```python
from build123d import *

# Parameters (mm, degrees)
CROQUIS1_W              = 50
CROQUIS1_H              = 46
CROQUIS1_W_2            = 44
CROQUIS1_H_2            = 40
SALIENTE_EXTRUIR1_DEPTH = 15
CROQUIS4_W              = 44
CROQUIS4_H              = 3
SALIENTE_EXTRUIR3_DEPTH = 10.7
CORTAR_EXTRUIR1_REACH   = 72.608
CROQUIS7_W              = 3
CROQUIS7_H              = 10.7
SALIENTE_EXTRUIR4_DEPTH = 10.7
SALIENTE_EXTRUIR5_DEPTH = 10.7
CORTAR_EXTRUIR2_REACH   = 72.778
CROQUIS9_R              = 6.65
CORTAR_EXTRUIR3_REACH   = 70.691
CROQUIS10_R             = 6.65
CROQUIS11_W             = 50
CROQUIS11_H             = 31.2
SALIENTE_EXTRUIR6_DEPTH = 2
CROQUIS12_W             = 3
CROQUIS12_H             = 12
SALIENTE_EXTRUIR7_DEPTH = 44
CORTAR_EXTRUIR4_REACH   = 62.537
CROQUIS13_R             = 2.5
REDONDEO1_R             = 2
CROQUIS15_W             = 2
CROQUIS15_H             = 10.7
SALIENTE_EXTRUIR8_DEPTH = 3
CROQUIS16_W             = 2.1
CROQUIS16_H             = 3.3
CORTAR_EXTRUIR5_DEPTH   = 50
CROQUIS17_W             = 2
CROQUIS17_H             = 10.7
SALIENTE_EXTRUIR9_DEPTH = 3
CORTAR_EXTRUIR6_REACH   = 69.968
CROQUIS18_W             = 4.444444444
CROQUIS18_H             = 21.2


with BuildPart() as part:
    # Croquis1 → Saliente-Extruir1 (new body)
    with BuildSketch(Plane(origin=(0, 0, 0), x_dir=(1, 0, 0), z_dir=(0, 1, 0))):
        with Locations((-22, -20)):
            Rectangle(CROQUIS1_W, CROQUIS1_H)
        with Locations((-22, -20)):
            Rectangle(CROQUIS1_W_2, CROQUIS1_H_2, mode=Mode.SUBTRACT)
    extrude(amount=SALIENTE_EXTRUIR1_DEPTH)

    # Croquis4 → Saliente-Extruir3 (add)
    with BuildSketch(Plane(origin=(0, 15, 0), x_dir=(1, 0, 0), z_dir=(0, 1, 0))):
        with Locations((-22, -41.5)):
            Rectangle(CROQUIS4_W, CROQUIS4_H)
    extrude(amount=SALIENTE_EXTRUIR3_DEPTH)

    # Croquis6 → Cortar-Extruir1 (cut, up to next)
    with BuildSketch(Plane.XY.offset(43), mode=Mode.PRIVATE) as cortar_extruir1_sk1:
        Polygon((-22, 24.7), (-11.85, 24.7), (-11.85, 16.7), (-32.15, 16.7), (-32.15, 24.7), align=None)
    cortar_extruir1_tool1 = extrude(cortar_extruir1_sk1.sketch, amount=-CORTAR_EXTRUIR1_REACH, mode=Mode.PRIVATE) & part.part
    add(cortar_extruir1_tool1.solids().sort_by_distance((-22, 20.7, 43))[0], mode=Mode.SUBTRACT)

    # Croquis7 → Saliente-Extruir4 (add)
    with BuildSketch(Plane.XY.offset(43)):
        with Locations((-45.5, 20.35)):
            Rectangle(CROQUIS7_W, CROQUIS7_H)
        with Locations((1.5, 20.35)):
            Rectangle(CROQUIS7_W, CROQUIS7_H)
    extrude(amount=-SALIENTE_EXTRUIR4_DEPTH)

    # Croquis8 → Saliente-Extruir5 (add)
    with BuildSketch(Plane(origin=(0, 15, 0), x_dir=(1, 0, 0), z_dir=(0, 1, 0))):
        Polygon((-47, -28.2), (-44, -28.2), (-44, 0), (0, 0), (0, -28.2), (3, -28.2), (3, 3), (-47, 3), align=None)
    extrude(amount=SALIENTE_EXTRUIR5_DEPTH)

    # Croquis9 → Cortar-Extruir2 (cut, up to next)
    with BuildSketch(Plane.ZY.offset(47), mode=Mode.PRIVATE) as cortar_extruir2_sk1:
        with Locations((7, 15.7)):
            Circle(CROQUIS9_R)
    cortar_extruir2_tool1 = extrude(cortar_extruir2_sk1.sketch, amount=-CORTAR_EXTRUIR2_REACH, mode=Mode.PRIVATE) & part.part
    add(cortar_extruir2_tool1.solids().sort_by_distance((-47, 15.7, 7))[0], mode=Mode.SUBTRACT)

    # Croquis10 → Cortar-Extruir3 (cut, up to next)
    with BuildSketch(Plane.ZY, mode=Mode.PRIVATE) as cortar_extruir3_sk1:
        with Locations((7, 15.7)):
            Circle(CROQUIS10_R)
    cortar_extruir3_tool1 = extrude(cortar_extruir3_sk1.sketch, amount=-CORTAR_EXTRUIR3_REACH, mode=Mode.PRIVATE) & part.part
    add(cortar_extruir3_tool1.solids().sort_by_distance((0, 15.7, 7))[0], mode=Mode.SUBTRACT)

    # Croquis11 → Saliente-Extruir6 (add)
    with BuildSketch(Plane(origin=(0, 25.7, 0), x_dir=(1, 0, 0), z_dir=(0, 1, 0))):
        with Locations((-22, -12.6)):
            Rectangle(CROQUIS11_W, CROQUIS11_H)
    extrude(amount=-SALIENTE_EXTRUIR6_DEPTH)

    # Croquis12 → Saliente-Extruir7 (add)
    with BuildSketch(Plane.ZY):
        with Locations((26.7, 17.7)):
            Rectangle(CROQUIS12_W, CROQUIS12_H)
    extrude(amount=SALIENTE_EXTRUIR7_DEPTH)

    # Croquis13 → Cortar-Extruir4 (cut, up to next)
    with BuildSketch(Plane(origin=(0, 0, 25.2), x_dir=(-1, 0, 0), z_dir=(0, 0, -1)), mode=Mode.PRIVATE) as cortar_extruir4_sk1:
        with Locations((6, 17.7)):
            Circle(CROQUIS13_R)
    cortar_extruir4_tool1 = extrude(cortar_extruir4_sk1.sketch, amount=-CORTAR_EXTRUIR4_REACH, mode=Mode.PRIVATE) & part.part
    # Croquis13 → Cortar-Extruir4 (cut, up to next)
    with BuildSketch(Plane(origin=(0, 0, 25.2), x_dir=(-1, 0, 0), z_dir=(0, 0, -1)), mode=Mode.PRIVATE) as cortar_extruir4_sk2:
        with Locations((38, 17.7)):
            Circle(CROQUIS13_R)
    cortar_extruir4_tool2 = extrude(cortar_extruir4_sk2.sketch, amount=-CORTAR_EXTRUIR4_REACH, mode=Mode.PRIVATE) & part.part
    add(cortar_extruir4_tool1.solids().sort_by_distance((-6, 17.7, 25.2))[0], mode=Mode.SUBTRACT)
    add(cortar_extruir4_tool2.solids().sort_by_distance((-38, 17.7, 25.2))[0], mode=Mode.SUBTRACT)

    # Redondeo1
    redondeo1_edges = [part.edges().sort_by_distance(p)[0] for p in [
        (-11.85, 16.7, 41.5),
        (-32.15, 16.7, 41.5),
    ]]
    fillet(redondeo1_edges, radius=REDONDEO1_R)

    # Croquis15 → Saliente-Extruir8 (add)
    with BuildSketch(Plane.ZY.offset(47)):
        with Locations((31.3, 20.35)):
            Rectangle(CROQUIS15_W, CROQUIS15_H)
    extrude(amount=-SALIENTE_EXTRUIR8_DEPTH)

    # Croquis16 → Cortar-Extruir5 (cut)
    with BuildSketch(Plane.ZY.offset(47)):
        with Locations((29.25, 13.35)):
            Rectangle(CROQUIS16_W, CROQUIS16_H)
    extrude(amount=-CORTAR_EXTRUIR5_DEPTH, mode=Mode.SUBTRACT)

    # Croquis17 → Saliente-Extruir9 (add)
    with BuildSketch(Plane(origin=(3, 0, 0), x_dir=(0, 0, -1), z_dir=(1, 0, 0))):
        with Locations((-31.3, 20.35)):
            Rectangle(CROQUIS17_W, CROQUIS17_H)
    extrude(amount=-SALIENTE_EXTRUIR9_DEPTH)

    # Croquis18 → Cortar-Extruir6 (cut, up to next)
    with BuildSketch(Plane.XZ.offset(-23.7), mode=Mode.PRIVATE) as cortar_extruir6_sk1:
        with Locations((-39.777777778, 12.6)):
            Rectangle(CROQUIS18_W, CROQUIS18_H)
    cortar_extruir6_tool1 = extrude(cortar_extruir6_sk1.sketch, amount=-CORTAR_EXTRUIR6_REACH, mode=Mode.PRIVATE) & part.part
    # Croquis18 → Cortar-Extruir6 (cut, up to next)
    with BuildSketch(Plane.XZ.offset(-23.7), mode=Mode.PRIVATE) as cortar_extruir6_sk2:
        with Locations((-30.888888889, 12.6)):
            Rectangle(CROQUIS18_W, CROQUIS18_H)
    cortar_extruir6_tool2 = extrude(cortar_extruir6_sk2.sketch, amount=-CORTAR_EXTRUIR6_REACH, mode=Mode.PRIVATE) & part.part
    # Croquis18 → Cortar-Extruir6 (cut, up to next)
    with BuildSketch(Plane.XZ.offset(-23.7), mode=Mode.PRIVATE) as cortar_extruir6_sk3:
        with Locations((-22, 12.6)):
            Rectangle(CROQUIS18_W, CROQUIS18_H)
    cortar_extruir6_tool3 = extrude(cortar_extruir6_sk3.sketch, amount=-CORTAR_EXTRUIR6_REACH, mode=Mode.PRIVATE) & part.part
    # Croquis18 → Cortar-Extruir6 (cut, up to next)
    with BuildSketch(Plane.XZ.offset(-23.7), mode=Mode.PRIVATE) as cortar_extruir6_sk4:
        with Locations((-13.111111111, 12.6)):
            Rectangle(CROQUIS18_W, CROQUIS18_H)
    cortar_extruir6_tool4 = extrude(cortar_extruir6_sk4.sketch, amount=-CORTAR_EXTRUIR6_REACH, mode=Mode.PRIVATE) & part.part
    # Croquis18 → Cortar-Extruir6 (cut, up to next)
    with BuildSketch(Plane.XZ.offset(-23.7), mode=Mode.PRIVATE) as cortar_extruir6_sk5:
        with Locations((-4.222222222, 12.6)):
            Rectangle(CROQUIS18_W, CROQUIS18_H)
    cortar_extruir6_tool5 = extrude(cortar_extruir6_sk5.sketch, amount=-CORTAR_EXTRUIR6_REACH, mode=Mode.PRIVATE) & part.part
    add(cortar_extruir6_tool1.solids().sort_by_distance((-39.777778, 23.7, 12.6))[0], mode=Mode.SUBTRACT)
    add(cortar_extruir6_tool2.solids().sort_by_distance((-30.888889, 23.7, 12.6))[0], mode=Mode.SUBTRACT)
    add(cortar_extruir6_tool3.solids().sort_by_distance((-22, 23.7, 12.6))[0], mode=Mode.SUBTRACT)
    add(cortar_extruir6_tool4.solids().sort_by_distance((-13.111111, 23.7, 12.6))[0], mode=Mode.SUBTRACT)
    add(cortar_extruir6_tool5.solids().sort_by_distance((-4.222222, 23.7, 12.6))[0], mode=Mode.SUBTRACT)


solid = part.part
```
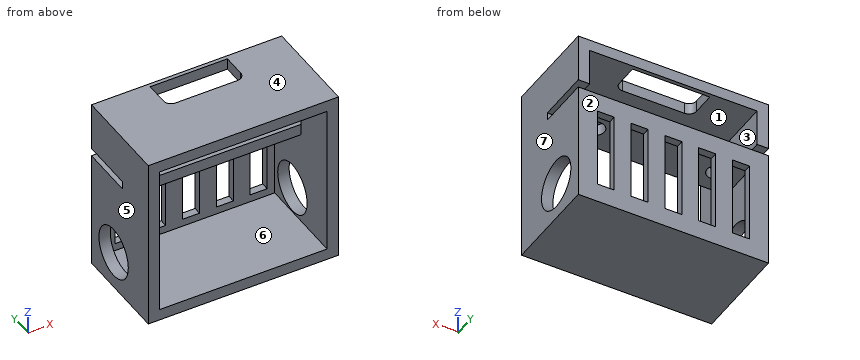
Design review of the part built by this model. Coordinates are the model's own, in mm. Face numbers are marked on the shaded views. A direction names the side the tool comes from. Round coordinates to 2 decimals unless told otherwise and drop trailing zeros. Order: outer loops, then holes, each group sorted by start corner. A loop starts at its lowest first (then second) coordinate and runs counter-clockwise, first axis right, second up. Notation, with made-up numbers: (22.5, -35) - (64.5, -35) arc R16 ccw to (64.5, -22) - close; hole circle Ø3 at (83, 56). An arc over 180 degrees is marked (long way). One line per question, with ' | ' between items.
Item 1: For P1, Ø7.5, axis at x = -29.5, z = 11.5, coming from the -Y side; P2, Ø3.5, axis at x = -27.5, z = 27, coming from the -Y side; P3, Ø3, axis at x = -19, y = 23, coming from the +Z side, all flat-tipped, find the tip position at first contact; note any pin that passes through.
Checks:
P1: y = 23.7 | P2: y = 11.7 | P3: z = 28.2
Item 2: Take a section at A-A, the plane z = 31.5. Write out the cut boundary in (x, y), then the cut area to 3 significant figures.
Checks:
outline: (-47, 0) - (-44, 0) - (-44, 25.7) - (-47, 25.7) - close; (0, 0) - (3, 0) - (3, 25.7) - (0, 25.7) - close | area: 154 mm²
Item 3: Take a section at C-C, the plane y = 5.25. Write out the cut boundary in (x, z), then the cut area to 3 significant figures.
Checks:
outline: (-47, -3) - (3, -3) - (3, 43) - (-47, 43) - close; hole (-44, 0) - (0, 0) - (0, 40) - (-44, 40) - close | area: 540 mm²
Item 4: Take a section at D-D, the plane y = 13. Write out the cut boundary in (x, z).
Checks:
outline: (-47, -3) - (3, -3) - (3, 0.92) - (0, 0.92) - (0, 0) - (-44, 0) - (-44, 0.92) - (-47, 0.92) - close; (-47, 13.08) - (-44, 13.08) - (-44, 25.2) - (0, 25.2) - (0, 13.08) - (3, 13.08) - (3, 28.2) - (-47, 28.2) - close; (-47, 30.3) - (-44, 30.3) - (-44, 40) - (0, 40) - (0, 30.3) - (3, 30.3) - (3, 43) - (-47, 43) - close
Item 5: Take a section at B-B, the plane x = -7.5. Write out the cut boundary in (y, z).
Checks:
outline: (0, -3) - (25.7, -3) - (25.7, 28.2) - (19.7, 28.2) - (19.7, 25.2) - (23.7, 25.2) - (23.7, 0) - (0, 0) - close; (0, 40) - (25.7, 40) - (25.7, 43) - (0, 43) - close; (11.7, 25.2) - (15.7, 25.2) - (15.7, 28.2) - (11.7, 28.2) - close
Item 6: Machinability: for the marked faces 1, 2 and 3, which of the approach directions +Z, -Z, +X, -X, +Y, -Y give a long, thin tool a straight path to every point of the face, cutting with its end or side? Answer none if there is none.
Checks:
face 1: +Y, -Y | face 2: +Z, -Z, +X, -X, +Y | face 3: -Y
Item 7: Wall thickness on line 1 (Z direction, x = -41.5, y = 22.25); line 2 (Z direction, x = -19, y = 11); line 3 (X direction, y = 8.5, z = 2): over which ranges is each line inside the solid? List them lowest first. Write a range as [from, to].
Checks:
line 1: [-3, 0], [25.2, 28.2], [40, 43] | line 2: [-3, 0], [40, 43] | line 3: [-47, -44], [0, 3]
Item 8: Draft analysis for pull direction X (two halves, no side actions). For the marked faces 4, 5, 6 and 7, state which applies: +X half, -X half, draft (parallel to the pull), parting line (faces both ways), or undercut.
Checks:
face 4: draft | face 5: -X half | face 6: undercut | face 7: +X half
